```python
from build123d import *

# Parameters (mm, degrees)
TAGLIO_ESTRUSIONE1_DEPTH      = 0.3
TAGLIO_ESTRUSIONE1_DEPTH_BACK = 0.3
TAGLIO_ESTRUSIONE2_DEPTH      = 0.3
TAGLIO_ESTRUSIONE2_DEPTH_BACK = 0.3
TAGLIO_ESTRUSIONE3_DEPTH      = 10.701
TAGLIO_ESTRUSIONE3_DEPTH_BACK = 10.701


with BuildPart() as part:
    # Schizzo1 → Rivoluzione1 (revolve)
    with BuildSketch(Plane.XY, mode=Mode.PRIVATE) as rivoluzione1_sk:
        with BuildLine():
            Line((14.2, 0), (14.2, 5.687947352))
            ThreePointArc((14.2, 5.687947352), (14.0596699, 6.035276538), (13.717449748, 6.187642766))
            Line((13.717449748, 6.187642766), (0, 6.666666667))
            Line((0, 6.666666667), (0, 9.0798475))
            Line((0, 9.0798475), (1.7, 9.0798475))
            Line((1.7, 9.0798475), (1.7, 10))
            Line((1.7, 10), (9.166666667, 10))
            Line((9.166666667, 10), (9.166666667, 12.380952381))
            Line((9.166666667, 12.380952381), (11, 12.380952381))
            Line((11, 12.380952381), (11, 20))
            Line((11, 20), (18, 13))
            Line((18, 13), (18, 10.25))
            Line((18, 10.25), (17.7, 10.25))
            Line((17.7, 10.25), (17.7, 0))
            Line((17.7, 0), (14.2, 0))
        make_face()
    revolve(rivoluzione1_sk.sketch.rotate(Axis((18, 0, 0), (-1, 0, 0)), 270), axis=Axis((18, 0, 0), (-1, 0, 0)))

    # Schizzo2 → Taglio-Estrusione1 (cut, two sides: drawn at the far end of the back side and taken through both)
    with BuildSketch(Plane(origin=(17.7, 0, 0), x_dir=(0, 0, -1), z_dir=(1, 0, 0)).offset(-TAGLIO_ESTRUSIONE1_DEPTH_BACK)):
        Polygon((-6.65, -4.7), (6.65, -4.7), (6.65, 2.3), (4.96521, 2.3), (6.17765, 4.4), (4.67654, 4.4), (2.71355, 1), (5.35, 1), (5.35, -3.4), (-5.35, -3.4), (-5.35, 1), (-2.71355, 1), (-4.67654, 4.4), (-6.17765, 4.4), (-4.96521, 2.3), (-6.65, 2.3), align=None)
    extrude(amount=TAGLIO_ESTRUSIONE1_DEPTH + TAGLIO_ESTRUSIONE1_DEPTH_BACK, mode=Mode.SUBTRACT)

    # Schizzo3 → Taglio-Estrusione2 (cut, two sides: drawn at the far end of the back side and taken through both)
    with BuildSketch(Plane(origin=(17.7, 0, 0), x_dir=(0, 0, -1), z_dir=(1, 0, 0)).offset(-TAGLIO_ESTRUSIONE2_DEPTH_BACK)):
        Polygon((-3.17543, 4.4), (0, -1.1), (3.17543, 4.4), (1.67432, 4.4), (0.65, 2.62583), (0.65, 8.2), (-0.65, 8.2), (-0.65, 2.62583), (-1.67432, 4.4), align=None)
    extrude(amount=TAGLIO_ESTRUSIONE2_DEPTH + TAGLIO_ESTRUSIONE2_DEPTH_BACK, mode=Mode.SUBTRACT)

    # Schizzo4 → Taglio-Estrusione3 (cut, two sides: drawn at the far end of the back side and taken through both)
    with BuildSketch(Plane(origin=(17.7, 0, 0), x_dir=(0, 0, -1), z_dir=(1, 0, 0)).offset(-TAGLIO_ESTRUSIONE3_DEPTH_BACK)):
        Polygon((-26, -15.011106999), (0, -30.022213998), (26, -15.011106999), (26, 15.011106999), (0, 30.022213998), (-26, 15.011106999), align=None)
        Polygon((-13, -7.505553499), (0, -15.011106999), (13, -7.505553499), (13, 7.505553499), (0, 15.011106999), (-13, 7.505553499), align=None, mode=Mode.SUBTRACT)
    extrude(amount=TAGLIO_ESTRUSIONE3_DEPTH + TAGLIO_ESTRUSIONE3_DEPTH_BACK, mode=Mode.SUBTRACT)


solid = part.part
```
The listing builds one solid part. Answer for the finished solid, in the listing's coordinates (mm). A direction names the side the tool comes from. Give positions to 0.01 mm unless a question says otherwise; leave off trailing zeros. Write each loop counter-clockwise with the first axis right and the second up, starting at its lowest first coordinate (ties: lowest second). Pieces come first, ordered by that corner, then holes. Notation, with made-up numbers: (36.25, 61.25) - (48.25, 61.25) arc R19 cw to (48.25, 76.25) - close; hole circle Ø8 at (-23.5, 62). An arc over 180 degrees is marked (long way). Use one line per item in the form item = value. Start each with the question number.
1) Find section C-C on x = 7.5. Determine the outline of the cut face in (y, z), plus the area to 3 significant figures.
2) The mould has two halves that part along Z. Classify faces 3 (the face through (14.2, 0, 0)), 4 (the face through (0.86, -5.52, -7.21)), 5 (the face through (14.45, -11.31, -6.41)): pulls with the +Z half, pulls with the -Z half, needs draft (parallel to the pull), parting line crosses it, or undercut.
3) Find section A-A on x = 10.5. Determine the outline of the cut face in (y, z), plus the area to 3 significant figures.
4) Consider line 1 along X through (y, z) = (-0.5, 8); line 2 along X through (y, z) = (-9, 2.75); line 3 along Y through (x, z) = (10.25, -1.25). Determine where each line is inside the solid, lowest interval first. Write a range as from..to.
5) Flat-ended cylindrical pins translate along their axes: pin 1 Ø1.5 at (x, z) = (13.5, -8) entering from +Y; pin 2 Ø10 at (y, z) = (-9, -7.5) entering from -X; pin 3 Ø7.5 at (y, z) = (1.5, -0.5) entering from +X; pin 4 Ø2 at (x, z) = (6, -7.5) entering from -Y. Find the tip coordinate at first contact, or state that the pin passes through.
6) Find section B-B on x = 15.5. Determine the outline of the cut face in (y, z).
7) A tool of negligible diameter and unlimited length cuts with its end or side. For faces 1 (the face through (18, 4, 10)), 2 (the face through (1.7, -8.1, 4.5)), from which of +Z, -Z, +X, -X, +Y, -Y can it reach the whole face along a straight path? Write none if from no direction.
Geometry results:
q1.outline = circle Ø20 at (0, 0); hole circle Ø12.81 at (0, 0)
q1.area = 185 mm2
q2.face_3 = undercut
q2.face_4 = parting line crosses it
q2.face_5 = pulls with the -Z half
q3.outline = circle Ø24.76 at (0, 0); hole circle Ø12.6 at (0, 0)
q3.area = 357 mm2
q4.line_1 = 0..17.7
q4.line_2 = 1.7..17.7
q4.line_3 = -12.32..-6.18, 6.18..12.32
q5.pin_1 = 10.83
q5.pin_2 = 0
q5.pin_3 = 17.7
q5.pin_4 = -7.6
q6.outline = (-15.01, 0) - (-7.51, -13) - (7.51, -13) - (15.01, 0) - (7.51, 13) - (-7.51, 13) - close
q7.face_1 = +Z, -Z, +X, +Y, -Y
q7.face_2 = -X
